Autodesk Inventor part; units mm, degrees
ref_plane "YZ Plane" through (0, 0, 0) normal (1, 0, 0) x (0, 1, 0)
ref_plane "XZ Plane" through (0, 0, 0) normal (0, 1, 0) x (-1, 0, 0)
ref_plane "XY Plane" through (0, 0, 0) normal (0, 0, 1) x (1, 0, 0)
sketch "Sketch1" plane through (0, 0, 0) normal (0, 0, 1) x (1, 0, 0)
  line L0 (-12.7, 0) -> (12.7, 0)
  line L1 (12.7, 0) -> (12.7, 25.4)
  line L2 (12.7, 25.4) -> (-12.7, 25.4)
  line L3 (-12.7, 25.4) -> (-12.7, 0)
  line L4 (-25.4, 25.4) -> (25.4, 25.4)
  line L5 (25.4, 25.4) -> (25.4, 76.2)
  line L6 (25.4, 76.2) -> (-25.4, 76.2)
  line L7 (-25.4, 76.2) -> (-25.4, 25.4)
  point P0 (0, 0)
  point P1 (0, 25.4)
  point P2 (0, 0)
  dimension "d0" = 25.4
  dimension "d1" = 50.8
  dimension "d2" = 25.4
  dimension "d3" = 50.8
extrude "Extrusion1" add sketch "Sketch1" along normal blind 3.175
sketch "Sketch2" plane through (0, 0, 3.175) normal (0, 0, 1) x (1, 0, 0)
  line L0 (-12.7, 0) -> (12.7, 0)
  line L1 (12.7, 0) -> (12.7, 25.4)
  line L2 (12.7, 25.4) -> (-12.7, 25.4)
  line L3 (-12.7, 25.4) -> (-12.7, 0)
  line L4 (25.4, 76.2) -> (25.4, 25.4)
  line L5 (-25.4, 76.2) -> (25.4, 76.2)
  line L6 (-25.4, 76.2) -> (25.4, 76.2)
  line L7 (25.4, 76.2) -> (25.4, 69.85)
  line L8 (25.4, 69.85) -> (-25.4, 69.85)
  line L9 (-25.4, 69.85) -> (-25.4, 76.2)
  line L10 (-12.7, 0) -> (-12.7, 25.4)
  line L11 (12.7, 25.4) -> (12.7, 0)
  line L12 (25.4, 25.4) -> (12.7, 25.4)
  line L13 (-12.7, 25.4) -> (-25.4, 25.4)
  line L14 (-12.7, 25.4) -> (-13.5255, 25.4)
  arc A0 (-12.7, 24.5745) -> (-13.5255, 25.4) centre (-13.5255, 24.5745) ccw
  line L15 (12.7, 25.4) -> (13.5255, 25.4)
  arc A1 (13.5255, 25.4) -> (12.7, 24.5745) centre (13.5255, 24.5745) ccw
  point P0 (0, 0)
  dimension "d17" = 6.35
  dimension "d19" = 0.8255
extrude "Extrusion2" add sketch "Sketch2" along normal blind 3.175 contours L3 L2 L1 L0 | L8 L9 L5 L4
fillet "Fillet1" radius 1.5875 2 edges at (12.7, 25.4, 1.5875) (-12.7, 25.4, 1.5875)
sketch "Sketch3" plane through (0, 0, 0) normal (0, 0, -1) x (-1, 0, 0)
  line L0 (12.7, 0) -> (-12.7, 0)
  point P0 (0, 0)
  point P1 (0, 6.35)
  point P2 (0, 19.05)
  point P3 (0, 0)
  dimension "d8" = 12.7
  dimension "d9" = 6.35
hole "Hole1" at (0, 6.35, 0) at (0, 19.05, 0) direction (0, 0, 1) diameter 5.1054 end through all
properties part number "gripper jaw extension"
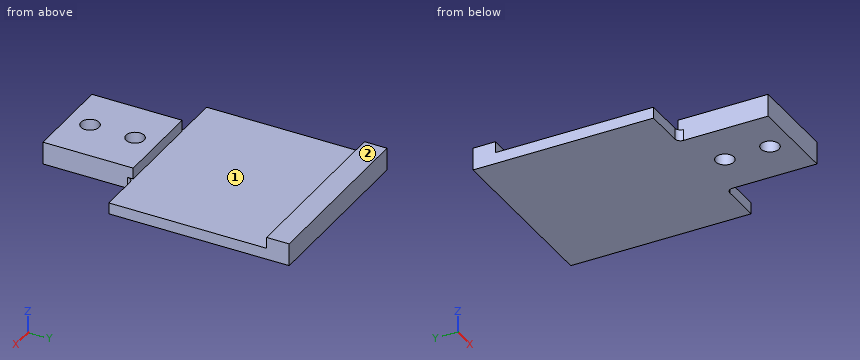
Model file for the job. Use its own axes, mm. Face numbers are marked on the shaded views. Coordinates: 2 decimals unless noted, no trailing zeros. Loops run counter-clockwise (first coordinate to the right, second up) from the corner with the lowest first, then second, coordinate; pieces in that order, holes last. Notation, with made-up numbers: (47, -23.75) -> (74, -23.75) arc R31 ccw to (74, 3.25) -> close; hole circle Ø4 at (11, 19). An arc over 180 degrees is marked (long way). Answer as a JSON object with one key per item and string values.
Q1. Cut at B-B (y = 19.05). List the corners of the cut face in (x, z), and give its area (3 significant figures).
Report:
{"outline": "(-12.7, 0) -> (-2.55, 0) -> (-2.55, 6.35) -> (-12.7, 6.35) -> close; (2.55, 0) -> (12.7, 0) -> (12.7, 6.35) -> (2.55, 6.35) -> close", "area": "129 mm2"}
Q2. Flat gauge pins, fed straight in: P1, Ø23, axis at x = -9.5, y = 43, coming from the +Z side (3 decimals); P2, Ø2.5, axis at x = 18.5, z = 2, coming from the -Y side; P3, Ø5, axis at x = -7.5, y = 33.5, coming from the -Z side; P4, Ø1.5, axis at y = 36.5, z = 4.5, coming from the +X side. Where does each tip first touch, or does it go through?
Report:
{"P1": "stops at z = 3.175", "P2": "stops at y = 25.4", "P3": "stops at z = 0", "P4": "passes through"}
Q3. Cut at A-A (z = 4). List the corners of the cut face in (x, y).
Report:
{"outline": "(-25.4, 69.85) -> (25.4, 69.85) -> (25.4, 76.2) -> (-25.4, 76.2) -> close; (-12.7, 0) -> (12.7, 0) -> (12.7, 25.4) -> (-12.7, 25.4) -> close; hole circle Ø5.11 at (0, 6.35); hole circle Ø5.11 at (0, 19.05)"}
Q4. Pull direction Y, two halves, no side cores. Call the marked faces 1 and 2: released by +Y, released by -Y, zero draft, split by the parting line, or undercut.
Report:
{"face 1": "undercut", "face 2": "zero draft"}
Q5. Cut at C-C (x = -8). List the corners of the cut face in (y, z) (3 decimals), and give its area (3 significant figures).
Report:
{"outline": "(0, 0) -> (76.2, 0) -> (76.2, 6.35) -> (69.85, 6.35) -> (69.85, 3.175) -> (25.4, 3.175) -> (25.4, 6.35) -> (0, 6.35) -> close", "area": "343 mm2"}
Q6. Probe probe 1 along Y at (x, z) = (0, 4); probe 2 along Y at (x, z) = (0, 2); probe 3 along X at (y, z) = (19.05, 4). List the from-to ranges inside material, lowest first.
Report:
{"probe 1": "y = 0 to 3.8, 8.9 to 16.5, 21.6 to 25.4, 69.85 to 76.2", "probe 2": "y = 0 to 3.8, 8.9 to 16.5, 21.6 to 76.2", "probe 3": "x = -12.7 to -2.55, 2.55 to 12.7"}
